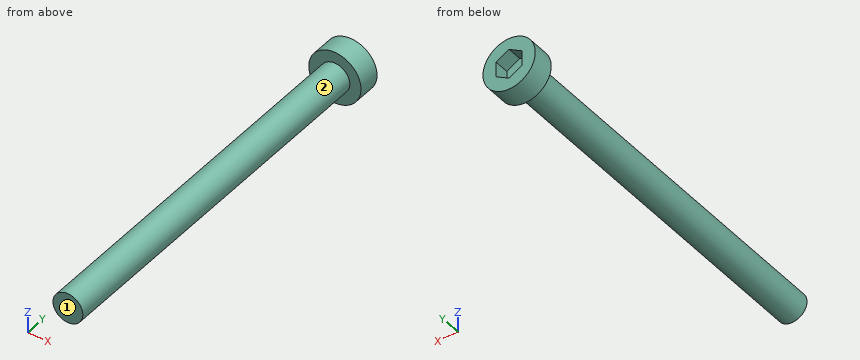
Autodesk Inventor part; units mm, degrees
ref_plane "YZ Plane" through (0, 0, 0) normal (1, 0, 0) x (0, 1, 0)
ref_plane "XZ Plane" through (0, 0, 0) normal (0, 1, 0) x (-1, 0, 0)
ref_plane "XY Plane" through (0, 0, 0) normal (0, 0, 1) x (1, 0, 0)
sketch "Sketch1" plane through (0, 0, 0) normal (0, 1, 0) x (-1, 0, 0)
  circle A0 centre (0, 0) radius 2
  dimension "d0" = 4
extrude "Extrusion1" add sketch "Sketch1" along normal blind 50
sketch "Sketch2" plane through (0, 50, 0) normal (0, 1, 0) x (1, 0, 0)
  circle A0 centre (0, 0) radius 3.5
  dimension "d3" = 7
extrude "Extrusion2" add sketch "Sketch2" along normal blind 3
sketch "Sketch3" plane through (0, 53, 0) normal (0, 1, 0) x (1, 0, 0)
  circle A0 centre (0, 0) radius 2
  line L0 (0, 2) -> (1.7321, 1)
  line L1 (1.7321, 1) -> (1.7321, -1)
  line L2 (1.7321, -1) -> (0, -2)
  line L3 (0, -2) -> (-1.7321, -1)
  line L4 (-1.7321, -1) -> (-1.7321, 1)
  line L5 (-1.7321, 1) -> (0, 2)
extrude "Extrusion3" cut sketch "Sketch3" against normal blind 2 contours L1 L2 L3 L4 L5 L0
properties part number "M4_shoulder_bolt"
Source: CAD feature listing. Evaluate the final solid. Frame: model axes, mm. Face numbers are marked on the shaded views. A direction names the side the tool comes from. Round coordinates to 2 decimals unless told otherwise and drop trailing zeros. Write each loop counter-clockwise with the first axis right and the second up, starting at its lowest first coordinate (ties: lowest second). Pieces come first, ordered by that corner, then holes. Notation, with made-up numbers: M 9,67.5 L 55,67.5 A23 ccw 55,97.5 Z; hole C 5,68 d4. An arc over 180 degrees is marked long. Use CSV: the item, a comma, the result in double quotes. Start each with the question number.
Q1. Line query: line 1 (Y direction, x = 1.25, z = 2.25); line 2 (X direction, y = 23, z = -1); line 3 (Y direction, x = 1, z = -0.5). Output: solid intervals per line, ascending. Write a range as from..to.
Q2. Cut plane C-C on y = 5. Output: boundary loops of the cut face in (x, z).
Q3. Cut plane A-A on z = 0. Output: boundary loops of the cut face in (x, y), plus the area to 3 significant figures.
Q4. First-contact query: P1, Ø1, axis at x = 0, z = 0.5, coming from the +Y side; P2, Ø1, axis at y = 52, z = 0.5, coming from the +X side; P3, Ø2, axis at x = -1, y = 44, coming from the +Z side; P4, Ø4, axis at x = 2, y = 44.5, coming from the -Z side. Flat tips, straight axial feed; report the tip coordinate or a pass-through.
Q5. Cut plane B-B on x = 2.5. Output: boundary loops of the cut face in (y, z), plus the area to 3 significant figures.
Q6. Access query for the marked faces 1 and 2. Directions: +Z, -Z, +X, -X, +Y, -Y. A direction counts if a zero-diameter tool reaches every point of the face in a straight line with its end or side. Return the directions, or none.
Results found:
1,line 1,"50..53"
1,line 2,"-1.73..1.73"
1,line 3,"0..51"
2,outline,"C 0,0 d4"
3,outline,"M -3.5,50 L -2,50 L -2,0 L 2,0 L 2,50 L 3.5,50 L 3.5,53 L 1.73,53 L 1.73,51 L -1.73,51 L -1.73,53 L -3.5,53 Z"
3,area,"214 mm^2"
4,P1,"y = 51"
4,P2,"x = 3.5"
4,P3,"z = 2"
4,P4,"z = -2"
5,outline,"M 50,-2.45 L 53,-2.45 L 53,2.45 L 50,2.45 Z"
5,area,"14.7 mm^2"
6,face 1,"+Z, -Z, +X, -X, -Y"
6,face 2,"-Y"
